from build123d import *
from build123d.topology import SkipClean

# Parameters (mm, degrees)
SKETCH1_R           = 25
BOSS_EXTRUDE1_DEPTH = 2.5
BOSS_EXTRUDE2_START = 10
BOSS_EXTRUDE2_DEPTH = 10
SKETCH4_R           = 12.5
CUT_EXTRUDE1_DEPTH  = 8.2
SKETCH6_R           = 2
CUT_EXTRUDE3_DEPTH  = 6
SKETCH8_R           = 2
CUT_EXTRUDE4_DEPTH  = 6


with BuildPart() as part:
    # Sketch1 → Boss-Extrude1 (new body)
    with BuildSketch(Plane.XY):
        Circle(SKETCH1_R)
    extrude(amount=BOSS_EXTRUDE1_DEPTH)

    # Sketch3 → Boss-Extrude2 (add)
    with SkipClean():  # the faces are left unmerged after this step: merging them gives an invalid solid
        with BuildSketch(Plane(origin=(0, 0, 0), x_dir=(-1, 0, 0), z_dir=(0, 0, -1)).offset(BOSS_EXTRUDE2_START)):
            with BuildLine():
                ThreePointArc((-3.021915591, -12.129221993), (-6.060912506, -18.245026612), (-11.704264354, -22.090952807))
                ThreePointArc((-11.704264354, -22.090952807), (0, -25), (11.704264354, -22.090952807))
                ThreePointArc((11.704264354, -22.090952807), (6.060912506, -18.245026612), (3.021915591, -12.129221993))
                ThreePointArc((3.021915591, -12.129221993), (0, -12.5), (-3.021915591, -12.129221993))
            make_face()
            with BuildLine():
                ThreePointArc((-24.983458502, 0.909286141), (-18.831112792, 3.873609106), (-12.01517217, 3.447555327))
                ThreePointArc((-12.01517217, 3.447555327), (-10.825317547, 6.25), (-8.993256579, 8.681666667))
                ThreePointArc((-8.993256579, 8.681666667), (-12.770200286, 14.371417506), (-13.279194148, 21.181666667))
                ThreePointArc((-13.279194148, 21.181666667), (-21.650635095, 12.5), (-24.983458502, 0.909286141))
            make_face()
            with BuildLine():
                ThreePointArc((12.01517217, 3.447555327), (18.831112792, 3.873609106), (24.983458502, 0.909286141))
                ThreePointArc((24.983458502, 0.909286141), (21.650635095, 12.5), (13.279194148, 21.181666667))
                ThreePointArc((13.279194148, 21.181666667), (12.770200286, 14.371417506), (8.993256579, 8.681666667))
                ThreePointArc((8.993256579, 8.681666667), (10.825317547, 6.25), (12.01517217, 3.447555327))
            make_face()
        extrude(amount=-BOSS_EXTRUDE2_DEPTH)

    # Sketch4 → Cut-Extrude1 (cut)
    with SkipClean():  # the faces are left unmerged after this step: merging them gives an invalid solid
        with BuildSketch(Plane(origin=(0, 0, 0), x_dir=(-1, 0, 0), z_dir=(0, 0, -1))):
            with Locations(Location((0, 0, 0), (0, 0, 180))):
                Circle(SKETCH4_R)
        extrude(amount=-CUT_EXTRUDE1_DEPTH, mode=Mode.SUBTRACT)

    # Sketch6 → Cut-Extrude3 (cut)
    with SkipClean():  # the faces are left unmerged after this step: merging them gives an invalid solid
        with BuildSketch(Plane(origin=(0, 0, -10), x_dir=(-1, 0, 0), z_dir=(0, 0, -1))):
            with Locations((16.237976321, 9.375)):
                Circle(SKETCH6_R)
            with Locations((0, -18.75)):
                Circle(SKETCH6_R)
            with Locations((-16.237976321, 9.375)):
                Circle(SKETCH6_R)
        extrude(amount=-CUT_EXTRUDE3_DEPTH, mode=Mode.SUBTRACT)

    # Sketch8 → Cut-Extrude4 (cut)
    with SkipClean():  # the faces are left unmerged after this step: merging them gives an invalid solid
        with BuildSketch(Plane(origin=(0, 0, 0), x_dir=(-1, 0, 0), z_dir=(0, 0, -1))):
            with Locations((-16.237976321, -9.375)):
                Circle(SKETCH8_R)
            with Locations((0, 18.75)):
                Circle(SKETCH8_R)
            with Locations((16.237976321, -9.375)):
                Circle(SKETCH8_R)
        extrude(amount=-CUT_EXTRUDE4_DEPTH, mode=Mode.SUBTRACT)


solid = part.part
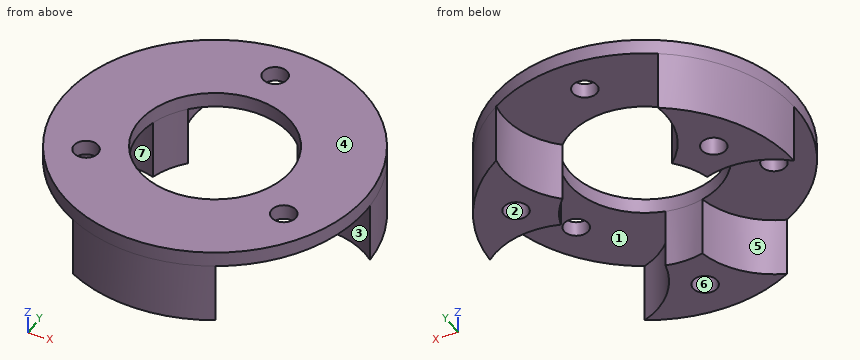
Could you check a few things on this model? Use its own coordinates, in mm. Face numbers are marked on the shaded views. A direction names the side the tool comes from. Give positions to 0.01 mm unless a question says otherwise; leave off trailing zeros. Order: outer loops, then holes, each group sorted by start corner. A loop starts at its lowest first (then second) coordinate and runs counter-clockwise, first axis right, second up. Notation, with made-up numbers: (-23.5, -1) - (-0.5, -1) arc R12 cw to (-0.5, 9) - close; hole circle Ø11 at (-9, 43). An arc over 180 degrees is marked (long way). Return JSON: item names as keys, results as strings. Group by question number.
Q1. Which directions (+Z, -Z, +X, -X, +Y, -Y) give clear straight access to the entire face, cutting with the end or side of a thin tool? Please do the marked faces 5, 6 and 7.
Q2. Will these pins go through, and if not, where does the flat tip stop? pin 1 Ø3 at (y, z) = (-4, -1) entering from -X; pin 2 Ø6.5 at (x, y) = (-16.24, -9.38) entering from +Z; pin 3 Ø13 at (x, y) = (3.5, 14.5) entering from -Z; pin 4 Ø3 at (x, y) = (-16.24, 9.38) entering from -Z.
Q3. Suppose I cut it at B-B, the plane z = -3. Please give me the cut outline in (x, y) (3 decimals), and give its area (3 significant figures).
Q4. Suppose I cut it at D-D, the plane x = -7. Please give me the cut outline in (y, z), and give its area (3 significant figures).
Q5. Suppose I cut it at A-A, the plane x = 0. Please give me the cut outline in (y, z), and give its area (4 significant figures).
Q6. Thinking about a two-plate mould opening in Y: for the marked faces 1, 2, 3 and 4, which applies, pulls with the +Y half, pulls with the -Y half, needs draft (parallel to the pull), parting line crosses it, or undercut?
Q7. Please list where these lines run through material, in increasing order: line 1 along Y through (x, z) = (0, 2); line 2 along X through (y, z) = (8, -8.25); line 3 along Z through (x, y) = (1, -19.5). Write a range as [from, to].
Q8. Suppose I cut it at C-C, the plane y = 0. Please give me the cut outline in (x, z), and give its area (3 significant figures).
Resolved:
{
 "1": {"face 5": "-Z, -X", "face 6": "-Z", "face 7": "-Z, -Y"},
 "2": {"pin 1": "stops at x = -24.83", "pin 2": "stops at z = 2.5", "pin 3": "stops at z = 0", "pin 4": "stops at z = -4"},
 "3": {"outline": "(-24.983, 0.909) arc R13.5 cw to (-12.015, 3.448) arc R12.5 cw to (-8.993, 8.682) arc R13.5 cw to (-13.279, 21.182) arc R25 ccw to start; (-11.704, -22.091) arc R25 ccw to (11.704, -22.091) arc R13.5 cw to (3.022, -12.129) arc R12.5 cw to (-3.022, -12.129) arc R13.5 cw to start; (8.993, 8.682) arc R12.5 cw to (12.015, 3.448) arc R13.5 cw to (24.983, 0.909) arc R25 ccw to (13.279, 21.182) arc R13.5 cw to start", "area": "481 mm2"},
 "4": {"outline": "(-24, -10) - (-19.22, -10) - (-19.22, 0) - (-10.36, 0) - (-10.36, 2.5) - (-24, 2.5) - close; (10.36, 0) - (24, 0) - (24, 2.5) - (10.36, 2.5) - close", "area": "116 mm2"},
 "5": {"outline": "(-25, -10) - (-20.75, -10) - (-20.75, -4) - (-16.75, -4) - (-16.75, -10) - (-12.5, -10) - (-12.5, 2.5) - (-25, 2.5) - close; (12.5, 0) - (16.75, 0) - (16.75, 2.5) - (12.5, 2.5) - close; (20.75, 0) - (25, 0) - (25, 2.5) - (20.75, 2.5) - close", "area": "153.5 mm2"},
 "6": {"face 1": "undercut", "face 2": "undercut", "face 3": "pulls with the -Y half", "face 4": "needs draft"},
 "7": {"line 1": "y = [-25, -12.5], [12.5, 16.75], [20.75, 25]", "line 2": "x = [-23.69, -17.69], [-14.79, -9.6], [9.6, 14.79], [17.69, 23.69]", "line 3": "z = [-4, 2.5]"},
 "8": {"outline": "(-25, 0) - (-12.5, 0) - (-12.5, 2.5) - (-25, 2.5) - close; (12.5, 0) - (25, 0) - (25, 2.5) - (12.5, 2.5) - close", "area": "62.5 mm2"}
}
